Verification items for the finished model (mm, model axes). A direction names the side the tool comes from. Coordinates: 2 decimals unless noted, no trailing zeros. Loops run counter-clockwise (first coordinate to the right, second up) from the corner with the lowest first, then second, coordinate; pieces in that order, holes last. Notation, with made-up numbers: (33.25, 13) - (43.25, 13) arc R28 ccw to (43.25, 47) - close; hole circle Ø11 at (62, 18.5). An arc over 180 degrees is marked (long way). One line per item, written item: value. Start each with the question number.
(1) Thickness scan on probe 1 along Y at (x, z) = (0, 58); probe 2 along X at (y, z) = (17, 41); probe 3 along X at (y, z) = (-19, 87). Record the ranges inside material, lowest first. Write a range as [from, to].
(2) Section check D-D (y = 17.5). Record the boundary of the cut face in (x, z).
(3) Gauge pin test, flat ends, axial feed: P1, Ø2, axis at y = -6, z = 20.5, coming from the +X side; P2, Ø8, axis at x = 30.5, z = 84.5, coming from the +Y side; P3, Ø12, axis at y = 39.5, z = 68.5, coming from the -X side; P4, Ø4, axis at x = 0, y = -35, coming from the +Z side. Record the tip position at first contact, or that the pin passes through.
(4) Section check A-A (z = 50). Record the boundary of the cut face in (x, y).
(5) Section check B-B (y = 0). Record the boundary of the cut face in (x, z), plus the area to 4 significant figures.
(6) Set-up check for faces 1 (the face through (-0.66, 44.885, 64.985)), 2 (the face through (0.54, 32.56, 49.3)), 3 (the face through (-7, 25, 7.5)): record each of +Z, -Z, +X, -X, +Y, -Y from which the full face is reachable in a straight line by a thin tool's end or side.
(7) Section check C-C (x = -18). Record the boundary of the cut face in (y, z), plus the area to 3 significant figures.
(8) Draft check along X on faces 4 (the face through (-8.67, -39.05, 49.3)), 5 (the face through (-27.813, 17.61, 49.3)), 6 (the face through (-18.34, -17.22, 100)). Enter one of: +X half, -X half, draft (parallel to the pull), parting line (faces both ways), or undercut.
```python
from build123d import *

# Parameters (mm, degrees)
SKETCH1_R              = 40
BODY_DEPTH             = 100
SKETCH3_R              = 25
MOTOR_CASING_DEPTH     = 246
SKETCH4_R              = 30
SLEW_BEARING_LIP_DEPTH = 7.5
BASE_START             = 30
SKETCH6_R              = 15
BASE_DEPTH             = 20
SKETCH5_R              = 2.5
SCREW_HOLES_DEPTH      = 119.74342103


with BuildPart() as part:
    # Sketch1 → body (new body)
    with BuildSketch(Plane.XY):
        Circle(SKETCH1_R)
    extrude(amount=BODY_DEPTH)

    # Sketch3 → motor casing (cut)
    with BuildSketch(Plane.XY):
        Circle(SKETCH3_R)
    extrude(amount=MOTOR_CASING_DEPTH, mode=Mode.SUBTRACT)

    # Sketch4 → slew bearing lip (cut)
    with BuildSketch(Plane.XY):
        Circle(SKETCH4_R)
    extrude(amount=SLEW_BEARING_LIP_DEPTH, mode=Mode.SUBTRACT)

    # Sketch6 → base (add)
    with BuildSketch(Plane(origin=(0, 0, 0), x_dir=(1, 0, 0), z_dir=(0, 1, 0)).offset(BASE_START)):
        with Locations(Location((0, -50, 0), (0, 0, 90))):
            Circle(SKETCH6_R)
    extrude(amount=BASE_DEPTH)

    # Sketch5 → screw holes (cut, through all)
    with BuildSketch(Plane(origin=(0, 0, 0), x_dir=(-1, 0, 0), z_dir=(0, 0, -1))):
        with Locations((0, 35)):
            Circle(SKETCH5_R)
        with Locations((30.310889132, 17.5)):
            Circle(SKETCH5_R)
        with Locations((30.310889132, -17.5)):
            Circle(SKETCH5_R)
        with Locations((0, -35)):
            Circle(SKETCH5_R)
        with Locations((-30.310889132, -17.5)):
            Circle(SKETCH5_R)
        with Locations((-30.310889132, 17.5)):
            Circle(SKETCH5_R)
    extrude(amount=-SCREW_HOLES_DEPTH, mode=Mode.SUBTRACT)


solid = part.part
```
Responses:
1. probe 1: y = [-40, -37.5], [-32.5, -25], [25, 32.5], [37.5, 50]
1. probe 2: x = [-36.21, -32.76], [-27.86, -18.33], [18.33, 27.86], [32.76, 36.21]
1. probe 3: x = [-35.2, -32.31], [-28.31, -16.25], [16.25, 28.31], [32.31, 35.2]
2. outline: (-35.97, 0) - (-32.81, 0) - (-32.81, 100) - (-35.97, 100) - close; (-27.81, 0) - (-24.37, 0) - (-24.37, 7.5) - (-17.85, 7.5) - (-17.85, 100) - (-27.81, 100) - close; (17.85, 7.5) - (24.37, 7.5) - (24.37, 0) - (27.81, 0) - (27.81, 100) - (17.85, 100) - close; (32.81, 0) - (35.97, 0) - (35.97, 100) - (32.81, 100) - close
3. P1: stops at x = 39.69
3. P2: stops at y = 29.96
3. P3: stops at x = -21.86
3. P4: passes through
4. outline: (-15, 37.08) arc R40 ccw (long way) to (15, 37.08) - (15, 50) - (-15, 50) - close; hole circle Ø5 at (-30.31, -17.5); hole circle Ø5 at (-30.31, 17.5); hole circle Ø50 at (0, 0); hole circle Ø5 at (0, -35); hole circle Ø5 at (0, 35); hole circle Ø5 at (30.31, -17.5); hole circle Ø5 at (30.31, 17.5)
5. outline: (-40, 0) - (-30, 0) - (-30, 7.5) - (-25, 7.5) - (-25, 100) - (-40, 100) - close; (25, 7.5) - (30, 7.5) - (30, 0) - (40, 0) - (40, 100) - (25, 100) - close
5. area: 2,925 mm²
6. face 1: +Y
6. face 2: +Z, -Z
6. face 3: -Z
7. outline: (-35.72, 0) - (-24, 0) - (-24, 7.5) - (-17.35, 7.5) - (-17.35, 100) - (-35.72, 100) - close; (17.35, 7.5) - (24, 7.5) - (24, 0) - (35.72, 0) - (35.72, 100) - (17.35, 100) - close
7. area: 3,570 mm²
8. face 4: parting line
8. face 5: undercut
8. face 6: draft
